Print and shaded views of the part. All mm, measured from the part's lowest x, y and z. Give positions to 0.01 mm unless a question says otherwise; leave off trailing zeros. Write each loop counter-clockwise with the first axis right and the second up, starting at its lowest first coordinate (ties: lowest second). Pieces come first, ordered by that corner, then holes. Notation, with made-up numbers: (43.25, 12.5) -> (61.25, 12.5) arc R14 cw to (61.25, 20.5) -> close; hole circle Ø4 at (24.25, 46.5). An arc over 180 degrees is marked (long way). Put each result on its own line as item: value.
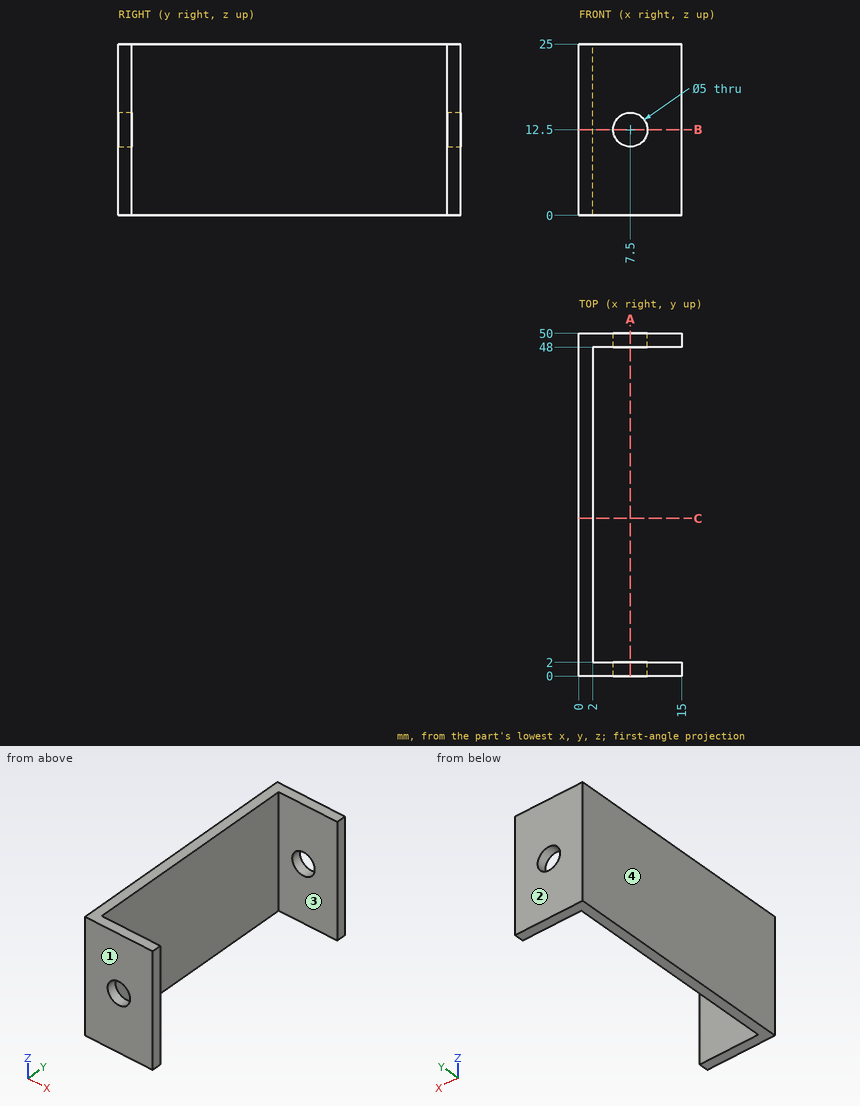
1) Slice it at B-B (z = 12.5). Write the cut outline in (x, y), plus the area to 3 significant figures.
Filled sheet:
outline: (0, 0) -> (5, 0) -> (5, 2) -> (2, 2) -> (2, 48) -> (5, 48) -> (5, 50) -> (0, 50) -> close; (10, 0) -> (15, 0) -> (15, 2) -> (10, 2) -> close; (10, 48) -> (15, 48) -> (15, 50) -> (10, 50) -> close
area: 132 mm2
2) Slice it at A-A (x = 7.5). Write the cut outline in (y, z).
Filled sheet:
outline: (0, 0) -> (2, 0) -> (2, 10) -> (0, 10) -> close; (0, 15) -> (2, 15) -> (2, 25) -> (0, 25) -> close; (48, 0) -> (50, 0) -> (50, 10) -> (48, 10) -> close; (48, 15) -> (50, 15) -> (50, 25) -> (48, 25) -> close
3) Slice it at C-C (y = 23). Write the cut outline in (x, z), plus the area to 3 significant figures.
Filled sheet:
outline: (0, 0) -> (2, 0) -> (2, 25) -> (0, 25) -> close
area: 50.0 mm2
4) Pull direction Y, two halves, no side cores. Call the marked faces 1, 2, 3 and 4: released by +Y, released by -Y, zero draft, split by the parting line, or undercut.
Filled sheet:
face 1: released by -Y
face 2: released by +Y
face 3: undercut
face 4: zero draft
5) Wall check: L1, parallel to Y at x = 14, z = 14.5; L2, parallel to X at y = 1.55, z = 12.5; L3, parallel to X at y = 29.5, z = 9.5. Give the ranges that are in metal, low to high.
Filled sheet:
L1: 0 to 2, 48 to 50
L2: 0 to 5, 10 to 15
L3: 0 to 2
6) Pin check, flat tips, straight feed: pin 1 (12.5 mm diameter, centred on y = 17.5, z = 12, fed in from +X); pin 2 (8 mm diameter, centred on x = 7.5, z = 12.5, fed in from +Y); pin 3 (4 mm diameter, centred on x = 7.5, z = 12.5, fed in from +Y). Stop position of each tip, or through.
Filled sheet:
pin 1: x = 2
pin 2: y = 50
pin 3: through
